Source: CAD feature listing. Evaluate the final solid. Frame: model axes, mm. A direction names the side the tool comes from. Give positions to 0.01 mm unless a question says otherwise; leave off trailing zeros. Loops run counter-clockwise (first coordinate to the right, second up) from the corner with the lowest first, then second, coordinate; pieces in that order, holes last. Notation, with made-up numbers: (83, 84.25) -> (115, 84.25) arc R20 cw to (115, 113.25) -> close; hole circle Ø5 at (62, -23.5). An arc over 180 degrees is marked (long way). Return JSON: item names as keys, results as strings. Group by question number.
(1) Cut plane B-B on y = 25. Return loops of the section in (x, z) (3 decimals), then the cut area to 3 significant figures.
(2) Cut plane C-C on y = 13.5. Return loops of the section in (x, z) (3 decimals).
(3) Draft query along Y for faces 4 (the face through (8, 38.45, -41)), 5 (the face through (45, 0, -47)), 6 (the face through (45, 16, 0)), 7 (the face through (76.835, 12, -3)). Return one class per face: released by +Y, released by -Y, zero draft, split by the parting line, or undercut.
(4) Cut plane A-A on x = 71. Return loops of the section in (y, z) (3 decimals), then the cut area to 3 significant figures.
(5) Pin query (flat end, axial travel): pin 1 (14 mm diameter, centred on x = 70.5, z = -17.5, fed in from +Y). Return the tip coordinate at first contact, or that it passes through.
(6) Ray query, line 1 (X direction, y = 14.5, z = -6.5) (3 decimals); line 2 (Z direction, x = 62.5, y = 9) (3 decimals); line 3 (X direction, y = 25, z = -33) (3 decimals). Return the intervals inside material, ascending. Write a range as from..to.
(7) Access query for faces 1 (the face through (7.99, 33.35, -38.78)), 2 (the face through (32, 27.02, -3)), 3 (the face through (70, 12, -49.53)). Directions: +Z, -Z, +X, -X, +Y, -Y. A direction counts if a zero-diameter tool reaches every point of the face in a straight line with its end or side. Return the directions, or none.
(8) Cut plane D-D on x = 39.5. Return loops of the section in (y, z) (3 decimals), then the cut area to 3 significant figures.
```python
from build123d import *

# Parameters (mm, degrees)
SKETCH1_W           = 92.075
SKETCH1_H           = 92.075
BOSS_EXTRUDE1_DEPTH = 32.1
SKETCH3_W           = 66.675
SKETCH3_H           = 81.915
CUT_EXTRUDE2_DEPTH  = 25.4
SKETCH4_R           = 1.905
BOSS_EXTRUDE2_DEPTH = 2.54
SKETCH4_3_R         = 1.905
BOSS_EXTRUDE3_DEPTH = 2.54
SKETCH8_W           = 2.142857143
SKETCH8_H           = 10
CUT_EXTRUDE4_DEPTH  = 7
BOSS_EXTRUDE5_DEPTH = 10.16
SKETCH11_W          = 12.7
SKETCH11_H          = 10.16
CUT_EXTRUDE5_DEPTH  = 7.62
SKETCH15_R          = 3.81
BOSS_EXTRUDE7_DEPTH = 3.81


with BuildPart() as part:
    # Sketch1 → Boss-Extrude1 (new body)
    with BuildSketch(Plane(origin=(0, 0, 0), x_dir=(1, 0, 0), z_dir=(0, 1, 0))):
        with Locations((46.0375, 46.0375)):
            Rectangle(SKETCH1_W, SKETCH1_H)
    extrude(amount=BOSS_EXTRUDE1_DEPTH)

    # Sketch3 → Cut-Extrude2 (cut)
    with BuildSketch(Plane(origin=(0, 32.1, 0), x_dir=(1, 0, 0), z_dir=(0, 1, 0))):
        with Locations((46.0375, 46.0375)):
            Rectangle(SKETCH3_W, SKETCH3_H)
    extrude(amount=-CUT_EXTRUDE2_DEPTH, mode=Mode.SUBTRACT)

    # Sketch4 → Boss-Extrude2 (add)
    with BuildSketch(Plane(origin=(0, 32.1, 0), x_dir=(1, 0, 0), z_dir=(0, 1, 0))):
        with Locations((8.405, 40.64)):
            Circle(SKETCH4_R)
    extrude(amount=BOSS_EXTRUDE2_DEPTH)

    # Sketch4<3> → Boss-Extrude3 (add)
    with BuildSketch(Plane(origin=(0, 32.1, 0), x_dir=(1, 0, 0), z_dir=(0, 1, 0))):
        with Locations((8.405, 40.64)):
            Circle(SKETCH4_3_R)
        with Locations((83.67, 40.64)):
            Circle(SKETCH4_3_R)
    extrude(amount=BOSS_EXTRUDE3_DEPTH)

    # Sketch8 → Cut-Extrude4 (cut)
    with BuildSketch(Plane.XY):
        with Locations((27.503571429, 22.02)):
            Rectangle(SKETCH8_W, SKETCH8_H)
        with Locations((31.567571429, 22.02)):
            Rectangle(SKETCH8_W, SKETCH8_H)
        with Locations((35.631571429, 22.02)):
            Rectangle(SKETCH8_W, SKETCH8_H)
    extrude(amount=-CUT_EXTRUDE4_DEPTH, mode=Mode.SUBTRACT)

    # Sketch10 → Boss-Extrude5 (add)
    with BuildSketch(Plane(origin=(0, 6.7, 0), x_dir=(1, 0, 0), z_dir=(0, 1, 0))):
        Polygon((61.595, 49.53), (79.375, 49.53), (79.375, 52.705), (58.42, 52.705), (58.42, 5.08), (61.595, 5.08), align=None)
    extrude(amount=BOSS_EXTRUDE5_DEPTH)

    # Sketch11 → Cut-Extrude5 (cut)
    with BuildSketch(Plane.XY):
        with Locations((70.485, 11.78)):
            Rectangle(SKETCH11_W, SKETCH11_H)
    extrude(amount=-CUT_EXTRUDE5_DEPTH, mode=Mode.SUBTRACT)

    # Sketch15 → Boss-Extrude7 (add)
    with BuildSketch(Plane(origin=(0, 34.64, 0), x_dir=(1, 0, 0), z_dir=(0, 1, 0))):
        with Locations((8.405, 40.64)):
            Circle(SKETCH15_R)
        with Locations((83.67, 40.64)):
            Circle(SKETCH15_R)
    extrude(amount=BOSS_EXTRUDE7_DEPTH)


solid = part.part
```
Answers:
{
 "1": {"outline": "(0, -92.075) -> (92.075, -92.075) -> (92.075, 0) -> (36.703, 0) -> (36.703, -5.08) -> (79.375, -5.08) -> (79.375, -86.995) -> (12.7, -86.995) -> (12.7, -5.08) -> (26.432, -5.08) -> (26.432, 0) -> (0, 0) -> close; (28.575, -5.08) -> (30.496, -5.08) -> (30.496, 0) -> (28.575, 0) -> close; (32.639, -5.08) -> (34.56, -5.08) -> (34.56, 0) -> (32.639, 0) -> close", "area": "2,980 mm²"},
 "2": {"outline": "(0, -92.075) -> (92.075, -92.075) -> (92.075, 0) -> (76.835, 0) -> (76.835, -5.08) -> (79.375, -5.08) -> (79.375, -49.53) -> (61.595, -49.53) -> (61.595, -5.08) -> (64.135, -5.08) -> (64.135, 0) -> (0, 0) -> close; hole (12.7, -86.995) -> (79.375, -86.995) -> (79.375, -52.705) -> (58.42, -52.705) -> (58.42, -5.08) -> (12.7, -5.08) -> close"},
 "3": {"face 4": "released by +Y", "face 5": "released by -Y", "face 6": "zero draft", "face 7": "undercut"},
 "4": {"outline": "(0, -92.075) -> (32.1, -92.075) -> (32.1, -86.995) -> (6.7, -86.995) -> (6.7, -52.705) -> (16.86, -52.705) -> (16.86, -49.53) -> (6.7, -49.53) -> (6.7, 0) -> (0, 0) -> close; (16.86, -5.08) -> (32.1, -5.08) -> (32.1, 0) -> (16.86, 0) -> close", "area": "856 mm²"},
 "5": {"pin 1": "y = 6.7"},
 "6": {"line 1": "0..12.7, 58.42..61.595, 79.375..92.075", "line 2": "-92.075..-86.995, -52.705..-49.53, -5.08..0", "line 3": "0..12.7, 79.375..92.075"},
 "7": {"face 1": "none", "face 2": "+Z", "face 3": "+Y"},
 "8": {"outline": "(0, -92.075) -> (32.1, -92.075) -> (32.1, -86.995) -> (6.7, -86.995) -> (6.7, -5.08) -> (32.1, -5.08) -> (32.1, 0) -> (0, 0) -> close", "area": "875 mm²"}
}
